Can you work these out from the model? Positions are in its coordinate system, mm. Face numbers are marked on the shaded views. A direction names the side the tool comes from. Coordinates: 2 decimals unless noted, no trailing zeros. Order: outer loops, then holes, each group sorted by start corner. A loop starts at its lowest first (then second) coordinate and runs counter-clockwise, first axis right, second up. Notation, with made-up numbers: (33, -29.75) -> (47, -29.75) arc R26 ccw to (47, 2.25) -> close; hole circle Ø6 at (-21.5, 66.25). An arc over 180 degrees is marked (long way). Answer in a Markdown table with one row per item. Add a question column.
1. Imagine slicing it at A-A on z = 14. Write out the boundary of the cut face in (x, y), plus the area to 3 significant figures.
2. We'd pull the mould along X, two halves only. Please class the marked faces 1, 2 and 3: pulls with the +X half, pulls with the -X half, needs draft (parallel to the pull), parting line crosses it, or undercut.
3. On a 3-axis mill with a long thin cutter (end or side, diameter ignored), from which of +Z, -Z, +X, -X, +Y, -Y can I reach the whole of each face in a straight line? I mean the marked faces 4, 5 and 6. Say none if no direction works.
4. Imagine slicing it at B-B on x = 132.8. Write out the boundary of the cut face in (y, z) (3 decimals).
5. If I drill on line 1 along Z through (x, y) = (127.5, 6.5); line 2 along X through (y, z) = (-0.25, 18.5); line 3 along Y through (x, z) = (8, 31.55) (3 decimals), over which ranges is the centre line in solid material (lowest first)? Write a range as [from, to].
6. Imagine slicing it at D-D on y = 0. State how many separate pieces and enclosed holes the cut face has, plus the area to 3 significant figures.
7. Will this pin go through, and if not, where does the flat tip stop? pin 1 (3 mm diameter, centred on x = 79, y = -3, fed in from +Z).
8. Imagine slicing it at C-C on y = -6.5. Write out the boundary of the cut face in (x, z).
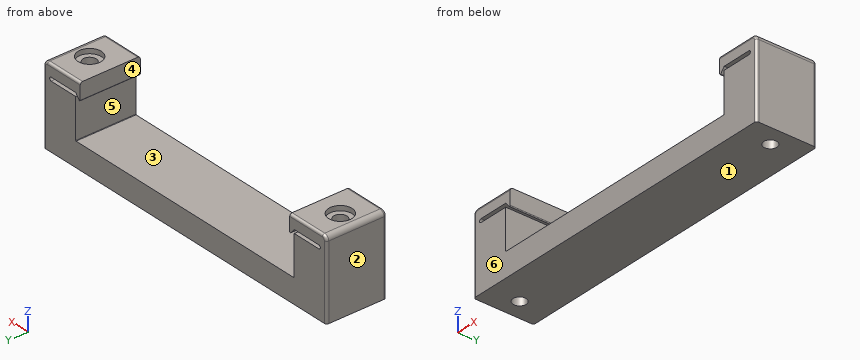
from build123d import *

# Parameters (mm, degrees)
F1_DEPTH       = 12.5
F4_D           = 5.5
F4_CBORE_D     = 9.75
F4_CBORE_DEPTH = 2
F5_R           = 2
F6_R           = 1


with BuildPart() as f1:
    # F0 (on Front) → F1 (new body, symmetric)
    with BuildSketch(Plane.XZ):
        with BuildLine():
            Line((0, 33), (0, 0))
            Line((0, 0), (70.4, 0))
            Line((70.4, 0), (70.4, 10))
            Line((70.4, 10), (16.2, 10))
            ThreePointArc((16.2, 10), (16.0585786438, 10.0585786438), (16, 10.2))
            Line((16, 10.2), (16, 26.6572023575))
            Line((16, 26.6572023575), (3.75, 26.6572023575))
            ThreePointArc((3.75, 26.6572023575), (3, 27.4072023575), (3.75, 28.1572023575))
            Line((3.75, 28.1572023575), (16, 28.1572023575))
            Line((16, 28.1572023575), (17.7201866671, 26.1071637171))
            ThreePointArc((17.7201866671, 26.1071637171), (18.052606043, 26.0180922138), (18.25, 26.3))
            Line((18.25, 26.3), (18.25, 33))
            Line((18.25, 33), (0, 33))
        make_face()
    extrude(amount=F1_DEPTH, both=True)

    # F4 (through all)
    with Locations(Plane.XY.offset(33)):
        with Locations((8, 0)):
            CounterBoreHole(F4_D / 2, F4_CBORE_D / 2, F4_CBORE_DEPTH)

    # F5
    f5_edges = [f1.edges().sort_by_distance(p)[0] for p in [
        (0, 0, 33),
    ]]
    fillet(f5_edges, radius=F5_R)

    # F6
    f6_edges = [f1.edges().sort_by_distance(p)[0] for p in [
        (10.125, -12.5, 33),
        (0.585786, -12.5, 32.414214),
        (0, -12.5, 15.5),
        (10.125, 12.5, 33),
        (0.585786, 12.5, 32.414214),
        (0, 12.5, 15.5),
    ]]
    fillet(f6_edges, radius=F6_R)

    # F7: F1 across plane


with BuildPart() as f1_1:
    add(f1.part)
    add(f1.part.mirror(Plane(origin=(70.4, 0, 5), x_dir=(0, 1, 0), z_dir=(1, 0, 0))))


solid = f1_1.part
Answers follow:
| question | item | result |
|---|---|---|
| 1 | outline | (0, -11.5) arc R1 ccw to (1, -12.5) -> (16, -12.5) -> (16, 12.5) -> (1, 12.5) arc R1 ccw to (0, 11.5) -> close; (124.8, -12.5) -> (139.8, -12.5) arc R1 ccw to (140.8, -11.5) -> (140.8, 11.5) arc R1 ccw to (139.8, 12.5) -> (124.8, 12.5) -> close; hole circle Ø5.5 at (8, 0); hole circle Ø5.5 at (132.8, 0) |
| 1 | area | 752 mm² |
| 2 | face 1 | needs draft |
| 2 | face 2 | pulls with the -X half |
| 2 | face 3 | undercut |
| 3 | face 4 | +Z, +Y, -Y |
| 3 | face 5 | +Y, -Y |
| 3 | face 6 | +Z, -Z, +X, -X, -Y |
| 4 | outline | (-12.5, 0) -> (-2.75, 0) -> (-2.75, 26.657) -> (-12.5, 26.657) -> close; (-12.5, 28.157) -> (-2.75, 28.157) -> (-2.75, 31) -> (-4.875, 31) -> (-4.875, 33) -> (-11.5, 33) arc R1 ccw to (-12.5, 32) -> close; (2.75, 0) -> (12.5, 0) -> (12.5, 26.657) -> (2.75, 26.657) -> close; (2.75, 28.157) -> (12.5, 28.157) -> (12.5, 32) arc R1 ccw to (11.5, 33) -> (4.875, 33) -> (4.875, 31) -> (2.75, 31) -> close |
| 5 | line 1 | z = [0, 26.66], [28.16, 33] |
| 5 | line 2 | x = [0, 5.26], [10.74, 16], [124.8, 130.06], [135.54, 140.8] |
| 5 | line 3 | y = [-12.5, -4.875], [4.875, 12.5] |
| 6 | separate pieces | 5 |
| 6 | enclosed holes | 0 |
| 6 | area | 1,770 mm² |
| 7 | pin 1 | stops at z = 10 |
| 8 | outline | (0, 0) -> (140.8, 0) -> (140.8, 31) arc R2 ccw to (138.8, 33) -> (122.55, 33) -> (122.55, 26.3) arc R0.3 ccw to (123.08, 26.11) -> (124.8, 28.16) -> (137.05, 28.16) arc R0.75 cw to (137.05, 26.66) -> (124.8, 26.66) -> (124.8, 10.2) arc R0.2 cw to (124.6, 10) -> (16.2, 10) arc R0.2 cw to (16, 10.2) -> (16, 26.66) -> (3.75, 26.66) arc R0.75 cw to (3.75, 28.16) -> (16, 28.16) -> (17.72, 26.11) arc R0.3 ccw to (18.25, 26.3) -> (18.25, 33) -> (2, 33) arc R2 ccw to (0, 31) -> close |
